from build123d import *

# Parameters (mm, degrees)
SKETCH1_R           = 3.4925
BASE_DEPTH          = 7.62
BOSS_EXTRUDE1_REACH = 52.684
SKETCH2_R           = 8.89
RIBS_DEPTH          = 2.54
EAR_1_DEPTH         = 3.556
EAR_2_DEPTH         = 3.556
EAR_3_DEPTH         = 3.556
SKETCH7_R           = 6.35
CUT_EXTRUDE5_DEPTH  = 51.683799656


with BuildPart() as part:
    # Sketch1 → Base (new body)
    with BuildSketch(Plane.XY):
        with BuildLine():
            Line((16.604256141, 33.560634381), (18.943472312, 23.673588932))
            ThreePointArc((18.943472312, 23.673588932), (20.401103388, 19.31706117), (22.619598737, 15.294338102))
            ThreePointArc((22.619598737, 15.294338102), (26.177171365, 7.766513011), (27.300719551, -0.483463539))
            ThreePointArc((27.300719551, -0.483463539), (28.309281475, -8.033336288), (31.510952034, -14.944709618))
            ThreePointArc((31.510952034, -14.944709618), (31.716980405, -21.01221602), (26.400801283, -23.943993837))
            Line((26.400801283, -23.943993837), (18.789002246, -23.590560073))
            ThreePointArc((18.789002246, -23.590560073), (14.751162948, -23.864172006), (10.879801534, -25.043820467))
            ThreePointArc((10.879801534, -25.043820467), (-2.658121922, -27.175308882), (-15.526424221, -22.460925535))
            ThreePointArc((-15.526424221, -22.460925535), (-19.339203493, -21.337609774), (-23.072841998, -22.701086061))
            ThreePointArc((-23.072841998, -22.701086061), (-30.228876792, -22.731059551), (-31.974558392, -15.791151184))
            Line((-31.974558392, -15.791151184), (-28.068905544, -6.994505511))
            ThreePointArc((-28.068905544, -6.994505511), (-27.342210837, -4.596155707), (-27.224673499, -2.092887453))
            ThreePointArc((-27.224673499, -2.092887453), (-20.610396453, 17.910180989), (-1.725707135, 27.250412105))
            ThreePointArc((-1.725707135, 27.250412105), (2.807988712, 29.118342831), (5.264931729, 33.361807717))
            ThreePointArc((5.264931729, 33.361807717), (10.854529977, 38.027365143), (16.604256141, 33.560634381))
        make_face()
        with Locations(Location((10.956281429, 32.224357143, 0), (0, 0, 180))):
            Circle(SKETCH1_R, mode=Mode.SUBTRACT)
        with Locations(Location((-26.67, -18.146340237, 0), (0, 0, 180))):
            Circle(SKETCH1_R, mode=Mode.SUBTRACT)
        with Locations(Location((26.67, -18.146340237, 0), (0, 0, 180))):
            Circle(SKETCH1_R, mode=Mode.SUBTRACT)
    extrude(amount=BASE_DEPTH)

    # Sketch2 → Boss-Extrude1 (add, up to next)
    with BuildSketch(Plane.XY.offset(8.255), mode=Mode.PRIVATE) as boss_extrude1_sk1:
        Circle(SKETCH2_R)
    boss_extrude1_tool1 = extrude(boss_extrude1_sk1.sketch, amount=-BOSS_EXTRUDE1_REACH, mode=Mode.PRIVATE) - part.part
    add(boss_extrude1_tool1.solids().sort_by_distance((0, 0, 8.255))[0])

    # Sketch3 → Ribs (cut)
    with BuildSketch(Plane.XY.offset(7.62)):
        with BuildLine():
            Line((-16.82050136, -8.986962316), (-9.437411961, -3.963488288))
            ThreePointArc((-9.437411961, -3.963488288), (-9.143653766, -3.575903337), (-9.144158406, -3.089574522))
            ThreePointArc((-9.144158406, -3.089574522), (-7.680637059, 5.845418599), (0.541368836, 9.636805696))
            ThreePointArc((0.541368836, 9.636805696), (1.010249912, 9.765904218), (1.305549154, 10.152316246))
            Line((1.305549154, 10.152316246), (4.752490825, 20.290380019))
            ThreePointArc((4.752490825, 20.290380019), (4.745775858, 20.799887499), (4.419461373, 21.191246438))
            ThreePointArc((4.419461373, 21.191246438), (2.971516318, 22.189265061), (1.673721066, 23.375988923))
            ThreePointArc((1.673721066, 23.375988923), (1.324970657, 23.584742075), (0.91851691, 23.584511061))
            ThreePointArc((0.91851691, 23.584511061), (-0.264361157, 23.321590055), (-1.468093727, 23.182464697))
            ThreePointArc((-1.468093727, 23.182464697), (-17.533671501, 15.236545944), (-23.160568555, -1.780458597))
            ThreePointArc((-23.160568555, -1.780458597), (-23.129900004, -3.436522013), (-23.291793081, -5.084938595))
            ThreePointArc((-23.291793081, -5.084938595), (-23.187534661, -5.603558506), (-22.770748598, -5.929328057))
            ThreePointArc((-22.770748598, -5.929328057), (-20.103253711, -7.131014955), (-17.77753644, -8.906013418))
            ThreePointArc((-17.77753644, -8.906013418), (-17.313377981, -9.116251065), (-16.82050136, -8.986962316))
        make_face()
        with BuildLine():
            Line((8.600175256, 18.982167319), (5.153233585, 8.844103546))
            ThreePointArc((5.153233585, 8.844103546), (5.151801602, 8.357776542), (5.444820248, 7.969632141))
            ThreePointArc((5.444820248, 7.969632141), (9.153474124, 3.061864703), (9.144158328, -3.089574805))
            ThreePointArc((9.144158328, -3.089574805), (9.143653829, -3.575903471), (9.437411961, -3.963488288))
            Line((9.437411961, -3.963488288), (16.820501249, -8.986962233))
            ThreePointArc((16.820501249, -8.986962233), (17.313378574, -9.116251013), (17.77753741, -8.906012507))
            ThreePointArc((17.77753741, -8.906012507), (20.193990454, -7.077426658), (22.972046166, -5.866898682))
            ThreePointArc((22.972046166, -5.866898682), (23.394092887, -5.548081357), (23.506917421, -5.031323638))
            ThreePointArc((23.506917421, -5.031323638), (23.275264524, -2.726844111), (23.225262219, -0.411290455))
            ThreePointArc((23.225262219, -0.411290455), (22.269437317, 6.607126953), (19.242940228, 13.011195948))
            ThreePointArc((19.242940228, 13.011195948), (17.372981423, 16.188369668), (15.914244764, 19.574114216))
            ThreePointArc((15.914244764, 19.574114216), (15.531519696, 20.001577905), (14.959105055, 20.040886782))
            ThreePointArc((14.959105055, 20.040886782), (12.216303466, 19.462229871), (9.413298568, 19.493341792))
            ThreePointArc((9.413298568, 19.493341792), (8.916062473, 19.381990041), (8.600175256, 18.982167319))
        make_face()
        with BuildLine():
            Line((7.151258875, -7.323488274), (14.534348232, -12.346962288))
            ThreePointArc((14.534348232, -12.346962288), (14.835546333, -12.757963676), (14.810381819, -13.26689313))
            ThreePointArc((14.810381819, -13.26689313), (13.998126604, -16.175763644), (13.888681178, -19.193926648))
            ThreePointArc((13.888681178, -19.193926648), (13.741882081, -19.709272424), (13.292122475, -20.00055849))
            ThreePointArc((13.292122475, -20.00055849), (11.242161258, -20.554754651), (9.255658504, -21.305275269))
            ThreePointArc((9.255658504, -21.305275269), (-2.455638263, -23.098740428), (-13.528106469, -18.883122199))
            ThreePointArc((-13.528106469, -18.883122199), (-13.763616748, -18.608952972), (-13.846300089, -18.257104539))
            ThreePointArc((-13.846300089, -18.257104539), (-14.078649652, -15.713760427), (-14.81038135, -13.266894204))
            ThreePointArc((-14.81038135, -13.266894204), (-14.83554649, -12.757964252), (-14.534348249, -12.346962301))
            Line((-14.534348249, -12.346962301), (-7.15125892, -7.323488332))
            ThreePointArc((-7.15125892, -7.323488332), (-6.682895541, -7.19252367), (-6.230707232, -7.37152571))
            ThreePointArc((-6.230707232, -7.37152571), (1.2e-08, -9.651999996), (6.230707236, -7.371525677))
            ThreePointArc((6.230707236, -7.371525677), (6.682895517, -7.192523649), (7.151258875, -7.323488274))
        make_face()
    extrude(amount=-RIBS_DEPTH, mode=Mode.SUBTRACT)

    # Sketch4 → Ear 1 (cut)
    with BuildSketch(Plane.XY.offset(7.62)):
        with BuildLine():
            Line((18.154678619, 27.007540298), (18.154678619, 40.040057117))
            Line((18.154678619, 40.040057117), (2.671053035, 40.040057117))
            Line((2.671053035, 40.040057117), (2.671053035, 29.001456211))
            ThreePointArc((2.671053035, 29.001456211), (9.820840691, 23.407165193), (18.154678619, 27.007540298))
        make_face()
    extrude(amount=-EAR_1_DEPTH, mode=Mode.SUBTRACT)

    # Sketch5 → Ear 2 (cut)
    with BuildSketch(Plane.XY.offset(7.62)):
        with BuildLine():
            Line((37.540663752, -9.512717098), (37.540663752, -27.850835624))
            Line((37.540663752, -27.850835624), (19.674041943, -27.850835624))
            Line((19.674041943, -27.850835624), (19.674041943, -23.631654346))
            ThreePointArc((19.674041943, -23.631654346), (19.201342522, -13.324384672), (28.789587575, -9.512717098))
            Line((28.789587575, -9.512717098), (37.540663752, -9.512717098))
        make_face()
    extrude(amount=-EAR_2_DEPTH, mode=Mode.SUBTRACT)

    # Sketch6 → Ear 3 (cut)
    with BuildSketch(Plane.XY.offset(7.62)):
        with BuildLine():
            Line((-29.241937643, -9.636508467), (-37.354784568, -9.636508467))
            Line((-37.354784568, -9.636508467), (-37.354784568, -30.196246958))
            Line((-37.354784568, -30.196246958), (-20.617156227, -30.196246958))
            Line((-20.617156227, -30.196246958), (-20.617156227, -25.655566183))
            ThreePointArc((-20.617156227, -25.655566183), (-20.457991369, -24.783962969), (-20.001042351, -24.024869295))
            ThreePointArc((-20.001042351, -24.024869295), (-19.189851268, -13.342230024), (-29.241937643, -9.636508467))
        make_face()
    extrude(amount=-EAR_3_DEPTH, mode=Mode.SUBTRACT)

    # Sketch7 → Cut-Extrude5 (cut, through all)
    with BuildSketch(Plane.XY.offset(8.255)):
        Circle(SKETCH7_R)
    extrude(amount=-CUT_EXTRUDE5_DEPTH, mode=Mode.SUBTRACT)


solid = part.part
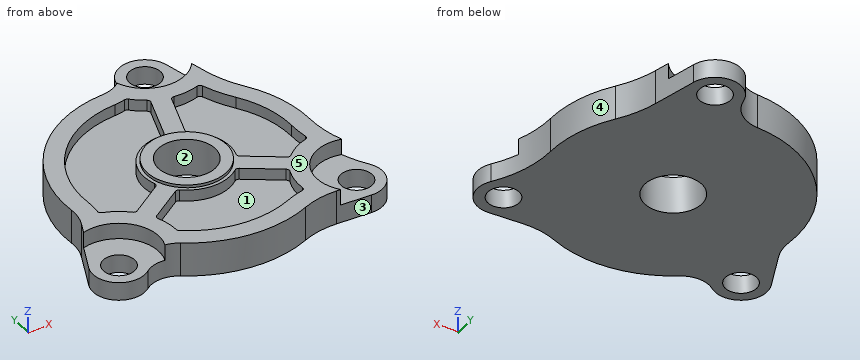
Input: part model. Units: mm. Frame: model coordinates. Face numbers are marked on the shaded views. A direction names the side the tool comes from. Give positions to 0.01 mm unless a question says otherwise; leave off trailing zeros. Write each loop counter-clockwise with the first axis right and the second up, starting at its lowest first coordinate (ties: lowest second). Pieces come first, ordered by that corner, then holes.
Q1. Pull-direction query (X, two-part tool) for the marked faces 3, 4 and 5; classes: pulls with the +X half, pulls with the -X half, needs draft (parallel to the pull), parting line crosses it, or undercut.
Q2. Material intervals for probe 1 along X at (y, z) = (8, 6.75); probe 2 along Z at (x, y) = (0.5, -16.5); probe 3 along Y at (x, z) = (13.5, 6.75), sorted ascending.
Q3. First-contact query: P1, Ø1, axis at y = -6, z = 7.5, coming from the -X side; P2, Ø12, axis at x = -22, y = -15.5, coming from the +Z side; P3, Ø8, axis at x = -6.5, y = -18, coming from the +Z side. Flat tips, straight axial feed; report the tip coordinate or a pass-through.
Q4. Set-up query: the marked faces 1 and 2. Return all of +Z, -Z, +X, -X, +Y, -Y with unobstructed straight access to the full face (end or side cutting, diameter ignored); none if empty.
Q5. Section A-A, the plane x = 12. Output: boundary loops of the cut face in (y, z), plus the area to 3 significant figures.
Q6. Section B-B, the plane z = 1. State how many separate pieces and enclosed holes the cut face has, plus the area to 3 significant figures.
Filled in:
1. face 3: undercut
1. face 4: pulls with the +X half
1. face 5: needs draft
2. probe 1: x = -26.11 to -21.81, -5.4 to 5.4, 21.81 to 26.11
2. probe 2: z = 0 to 5.08
2. probe 3: y = -24.14 to -19.92, -11.64 to -6.73, 19.65 to 23.71
3. P1: stops at x = -27.86
3. P2: stops at z = 7.62
3. P3: stops at z = 5.08
4. face 1: +Z
4. face 2: +Z, -Z
5. outline: (-24.6, 0) - (28.89, 0) - (28.89, 4.06) - (23.4, 4.06) - (23.4, 7.62) - (19.44, 7.62) - (19.44, 5.08) - (-5.71, 5.08) - (-5.71, 7.62) - (-10.62, 7.62) - (-10.62, 5.08) - (-20.32, 5.08) - (-20.32, 7.62) - (-24.6, 7.62) - close; (35.56, 0) - (37.93, 0) - (37.93, 4.06) - (35.56, 4.06) - close
5. area: 309 mm2
6. separate pieces: 1
6. enclosed holes: 4
6. area: 2,560 mm2
